Source: CAD feature listing. Evaluate the final solid. Frame: model axes, mm. Face numbers are marked on the shaded views. A direction names the side the tool comes from. Round coordinates to 2 decimals unless told otherwise and drop trailing zeros. Order: outer loops, then holes, each group sorted by start corner. A loop starts at its lowest first (then second) coordinate and runs counter-clockwise, first axis right, second up. Notation, with made-up numbers: M 85,7.25 L 121,7.25 A16 cw 121,15.25 Z; hole C -27.5,-0.5 d6. An arc over 180 degrees is marked long. Answer in a Markdown table with one row per item. Add a question column.
```python
from build123d import *

# Parameters (mm, degrees)
BOSS_EXTRUDE1_DEPTH = 2.54
SKETCH2_W           = 203.2
SKETCH2_H           = 101.6
BOSS_EXTRUDE2_DEPTH = 99.06
CHAMFER2_SIZE       = 45.56
CHAMFER3_SIZE       = 4.92
CHAMFER4_SIZE       = 4.92
FILLET1_R           = 4.92
FILLET3_R           = 4.92
CHAMFER5_SIZE       = 10
FILLET4_R           = 10
SKETCH4_R           = 25.4
CUT_EXTRUDE1_DEPTH  = 12.7
SKETCH5_R           = 3.81
BOSS_EXTRUDE3_DEPTH = 7.62
SKETCH7_R           = 2.032
BOSS_EXTRUDE4_DEPTH = 5.08
SKETCH8_R           = 19.05
CUT_EXTRUDE2_DEPTH  = 3.81
SKETCH9_W           = 185.084164058
SKETCH9_H           = 84.996684453
CUT_EXTRUDE3_DEPTH  = 64.77
SKETCH10_W          = 37.50506442
SKETCH10_H          = 86.993995576
CUT_EXTRUDE4_DEPTH  = 29.21
SKETCH11_W          = 25.743121139
SKETCH11_H          = 84.996684453
CUT_EXTRUDE5_DEPTH  = 19.05


with BuildPart() as part:
    # Sketch1 → Boss-Extrude1 (new body)
    with BuildSketch(Plane(origin=(0, 0, 0), x_dir=(1, 0, 0), z_dir=(0, 1, 0))):
        with BuildLine():
            Line((14.508978226, 50.8), (22.487986765, 42.820991461))
            Line((22.487986765, 42.820991461), (37.396380497, 42.820991461))
            Line((37.396380497, 42.820991461), (37.396380497, 38.724667236))
            Line((37.396380497, 38.724667236), (49.657488857, 38.724667236))
            Line((49.657488857, 38.724667236), (49.657488857, 42.820991461))
            Line((49.657488857, 42.820991461), (57.422857485, 42.820991461))
            add(Edge.make_bspline(
                [(57.422857485, 42.820991461), (65.475972879, 42.629610348), (68.662206814, 50.8)],
                knots=[0, 0, 0, 1, 1, 1], degree=2))
            Line((68.662206814, 50.8), (101.6, 50.8))
            Line((101.6, 50.8), (101.6, -50.8))
            Line((101.6, -50.8), (68.662206814, -50.8))
            add(Edge.make_bspline(
                [(57.422857485, -42.820991461), (65.475972879, -42.629610348), (68.662206814, -50.8)],
                knots=[0, 0, 0, 1, 1, 1], degree=2))
            Line((57.422857485, -42.820991461), (49.657488857, -42.820991461))
            Line((49.657488857, -42.820991461), (49.657488857, -38.724667236))
            Line((49.657488857, -38.724667236), (37.396380497, -38.724667236))
            Line((37.396380497, -38.724667236), (37.396380497, -42.820991461))
            Line((37.396380497, -42.820991461), (22.487986765, -42.820991461))
            Line((22.487986765, -42.820991461), (14.508978226, -50.8))
            Line((14.508978226, -50.8), (-101.6, -50.8))
            Line((-101.6, -50.8), (-101.6, 50.8))
            Line((-101.6, 50.8), (14.508978226, 50.8))
        make_face()
    extrude(amount=BOSS_EXTRUDE1_DEPTH)

    # Sketch2 → Boss-Extrude2 (add)
    with BuildSketch(Plane(origin=(0, 2.54, 0), x_dir=(1, 0, 0), z_dir=(0, 1, 0))):
        Rectangle(SKETCH2_W, SKETCH2_H)
    extrude(amount=BOSS_EXTRUDE2_DEPTH)

    # Chamfer2
    chamfer2_edges = [part.edges().sort_by_distance(p)[0] for p in [
        (-101.6, 101.6, 0),
    ]]
    chamfer(chamfer2_edges, length=CHAMFER2_SIZE)

    # Chamfer3
    chamfer3_edges = [part.edges().sort_by_distance(p)[0] for p in [
        (101.6, 101.6, 0),
    ]]
    chamfer(chamfer3_edges, length=CHAMFER3_SIZE)

    # Chamfer4
    chamfer4_edges = [part.edges().sort_by_distance(p)[0] for p in [
        (-101.6, 0, 0),
    ]]
    chamfer(chamfer4_edges, length=CHAMFER4_SIZE)

    # Fillet1
    fillet1_edges = [part.edges().sort_by_distance(p)[0] for p in [
        (20.32, 101.6, -50.8),
        (20.32, 101.6, 50.8),
    ]]
    fillet(fillet1_edges, radius=FILLET1_R)

    # Fillet3
    fillet3_edges = [part.edges().sort_by_distance(p)[0] for p in [
        (101.6, 48.34, 50.8),
        (101.6, 48.34, -50.8),
    ]]
    fillet(fillet3_edges, radius=FILLET3_R - 0.0001)  # a hair under: the kernel refuses the full size

    # Chamfer5
    chamfer5_edges = [part.edges().sort_by_distance(p)[0] for p in [
        (-101.6, 30.48, -50.8),
        (-101.6, 30.48, 50.8),
    ]]
    chamfer(chamfer5_edges, length=CHAMFER5_SIZE)

    # Fillet4
    fillet4_edges = [part.edges().sort_by_distance(p)[0] for p in [
        (-101.6, 4.92, 0),
        (-101.6, 56.04, 0),
        (-101.6, 30.48, 40.8),
        (-101.6, 30.48, -40.8),
        (-91.6, 33.02, -50.8),
        (-91.6, 33.02, 50.8),
    ]]
    fillet(fillet4_edges, radius=FILLET4_R)

    # Sketch4 → Cut-Extrude1 (cut)
    with BuildSketch(Plane.XY.offset(50.8)):
        with Locations((43.526934677, 7.68715588)):
            Circle(SKETCH4_R)
    cut_extrude1 = extrude(amount=-CUT_EXTRUDE1_DEPTH, mode=Mode.SUBTRACT)

    # Mirror1: Cut-Extrude1 across plane
    add(cut_extrude1.mirror(Plane.XY), mode=Mode.SUBTRACT)

    # Sketch5 → Boss-Extrude3 (add)
    with BuildSketch(Plane.XY.offset(38.1)):
        with Locations((43.526934677, 7.68715588)):
            Circle(SKETCH5_R)
    boss_extrude3 = extrude(amount=BOSS_EXTRUDE3_DEPTH)

    # Mirror2: Boss-Extrude3 across plane
    add(boss_extrude3.mirror(Plane.XY))

    # Sketch7 → Boss-Extrude4 (add)
    with BuildSketch(Plane.XY.offset(45.72)):
        with Locations((43.526934677, 7.68715588)):
            Circle(SKETCH7_R)
    boss_extrude4 = extrude(amount=BOSS_EXTRUDE4_DEPTH)

    # Mirror3: Boss-Extrude4 across plane
    add(boss_extrude4.mirror(Plane.XY))

    # Sketch8 → Cut-Extrude2 (cut)
    with BuildSketch(Plane.XZ):
        with Locations(Location((-57.478175649, 0, 0), (0, 0, 270))):
            Circle(SKETCH8_R)
    extrude(amount=-CUT_EXTRUDE2_DEPTH, mode=Mode.SUBTRACT)

    # Sketch9 → Cut-Extrude3 (cut)
    with BuildSketch(Plane(origin=(0, 101.6, 0), x_dir=(1, 0, 0), z_dir=(0, 1, 0))):
        with Locations((39.502375542, 0.665770374)):
            Rectangle(SKETCH9_W, SKETCH9_H)
    extrude(amount=-CUT_EXTRUDE3_DEPTH, mode=Mode.SUBTRACT)

    # Sketch10 → Cut-Extrude4 (cut)
    with BuildSketch(Plane(origin=(0, 36.83, 0), x_dir=(1, 0, 0), z_dir=(0, 1, 0))):
        with Locations((101.529982082, -0.332885187)):
            Rectangle(SKETCH10_W, SKETCH10_H)
    extrude(amount=-CUT_EXTRUDE4_DEPTH, mode=Mode.SUBTRACT)

    # Sketch11 → Cut-Extrude5 (cut)
    with BuildSketch(Plane(origin=(0, 36.83, 0), x_dir=(1, 0, 0), z_dir=(0, 1, 0))):
        with Locations((81.002062208, 0.665770374)):
            Rectangle(SKETCH11_W, SKETCH11_H)
    extrude(amount=-CUT_EXTRUDE5_DEPTH, mode=Mode.SUBTRACT)


solid = part.part
```
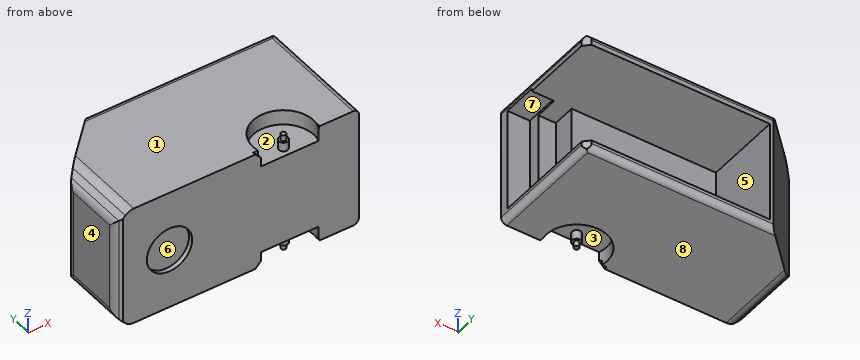
(1) Pin query (flat end, axial travel): pin 1 (10 mm diameter, centred on x = -63.5, z = 3.5, fed in from +Y); pin 2 (1 mm diameter, centred on x = 11, z = 29.5, fed in from +Y); pin 3 (9.5 mm diameter, centred on y = 26, z = -7.5, fed in from +X). Return the tip coordinate at first contact, or that it passes through.
(2) Line query: line 1 (Z direction, x = 68, y = 42); line 2 (Y direction, x = -34, z = -8.5); line 3 (X direction, y = 2, z = 0). Output: solid intervals per line, ascending. Write a range as from..to.
(3) Cut plane D-D (z = -17). Return loops of the section in (x, y).
(4) Access query for the marked faces 5, 6, 7 and 8. Directions: +Z, -Z, +X, -X, +Y, -Y. A direction counts if a zero-diameter tool reaches every point of the face in a straight line with its end or side. Return the directions, or none.
(5) Cut plane A-A (z = 0). Return loops of the section in (x, y), and give its area (3 significant figures).
(6) Cut plane C-C (y = 88.5). Return loops of the section in (x, z).
(7) Cut plane B-B (x = -11). Return loops of the section in (y, z).
(8) Draft query along X for the marked faces 1, 2, 3 and 4. Return one class per face: +X half, -X half, draft (parallel to the pull), parting line (faces both ways), or undercut.
Answer list:
| question | item | result |
|---|---|---|
| 1 | pin 1 | y = 99.14 |
| 1 | pin 2 | y = 36.83 |
| 1 | pin 3 | x = 68.13 |
| 2 | line 1 | -50.8..-43.16, 41.83..50.8 |
| 2 | line 2 | 0..36.83 |
| 2 | line 3 | -98.68..-76.53, -38.43..101.6 |
| 3 | outline | M -101.6,9.06 A10 ccw -98.67,1.99 L -96.68,0 L -66.07,0 L -66.07,3.81 L -48.88,3.81 L -48.88,0 L 101.6,0 L 101.6,7.62 L 82.78,7.62 L 82.78,17.78 L 68.13,17.78 L 68.13,36.83 L -53.04,36.83 L -53.04,101.6 L -56.04,101.6 L -98.67,58.97 A10 ccw -101.6,51.9 Z |
| 4 | face 5 | +X, +Y |
| 4 | face 6 | -Y |
| 4 | face 7 | +X |
| 4 | face 8 | -Z, +X, -X, +Y, -Y |
| 5 | outline | M -101.6,9.06 A10 ccw -98.67,1.99 L -96.68,0 L -76.53,0 L -76.53,3.81 L -38.43,3.81 L -38.43,0 L 101.6,0 L 101.6,7.62 L 82.78,7.62 L 82.78,17.78 L 68.13,17.78 L 68.13,36.83 L -53.04,36.83 L -53.04,101.6 L -56.04,101.6 L -98.67,58.97 A10 ccw -101.6,51.9 Z |
| 5 | area | 8,600 mm² |
| 6 | outline | M -69.14,-50.8 L 96.68,-50.8 A4.92 ccw 101.6,-45.88 L 101.6,-43.16 L -53.04,-43.16 L -53.04,41.83 L 101.6,41.83 L 101.6,45.88 A4.92 ccw 96.68,50.8 L -69.14,50.8 Z |
| 7 | outline | M 0,-50.8 L 96.68,-50.8 A4.92 ccw 101.6,-45.88 L 101.6,-43.16 L 36.83,-43.16 L 36.83,41.83 L 101.6,41.83 L 101.6,45.88 A4.92 ccw 96.68,50.8 L 0,50.8 Z |
| 8 | face 1 | draft |
| 8 | face 2 | undercut |
| 8 | face 3 | undercut |
| 8 | face 4 | -X half |
